```python
from build123d import *

# Parameters (mm, degrees)
SKETCH1_W           = 282.575
SKETCH1_H           = 384.175
SKETCH1_R           = 6.35
SKETCH1_R_2         = 1.5875
SKETCH1_W_2         = 127
SKETCH1_H_2         = 127
BOSS_EXTRUDE1_DEPTH = 2.54


with BuildPart() as part:
    # Sketch1 → Boss-Extrude1 (new body)
    with BuildSketch(Plane.XY):
        Rectangle(SKETCH1_W, SKETCH1_H)
        with Locations((-128.5875, 166.6875)):
            Circle(SKETCH1_R, mode=Mode.SUBTRACT)
        with Locations((-128.5875, -1.5875)):
            Circle(SKETCH1_R, mode=Mode.SUBTRACT)
        with Locations((-128.5875, -169.8625)):
            Circle(SKETCH1_R, mode=Mode.SUBTRACT)
        with Locations((128.5875, -1.5875)):
            Circle(SKETCH1_R, mode=Mode.SUBTRACT)
        with Locations((128.5875, 166.6875)):
            Circle(SKETCH1_R, mode=Mode.SUBTRACT)
        with Locations((128.5875, -169.8625)):
            Circle(SKETCH1_R, mode=Mode.SUBTRACT)
        with Locations((-80.175152311, 147.376386757)):
            Circle(SKETCH1_R_2, mode=Mode.SUBTRACT)
        with Locations((-80.175152311, 71.176386757)):
            Circle(SKETCH1_R_2, mode=Mode.SUBTRACT)
        with Locations((-80.175152311, -5.023613243)):
            Circle(SKETCH1_R_2, mode=Mode.SUBTRACT)
        with Locations((79.970650499, -5.395164494)):
            Circle(SKETCH1_R_2, mode=Mode.SUBTRACT)
        with Locations((79.970650499, 70.804835506)):
            Circle(SKETCH1_R_2, mode=Mode.SUBTRACT)
        with Locations((79.970650499, 147.004835506)):
            Circle(SKETCH1_R_2, mode=Mode.SUBTRACT)
        with Locations((-0.006402311, 49.2125)):
            Rectangle(SKETCH1_W_2, SKETCH1_H_2, mode=Mode.SUBTRACT)
    extrude(amount=BOSS_EXTRUDE1_DEPTH)


solid = part.part
```
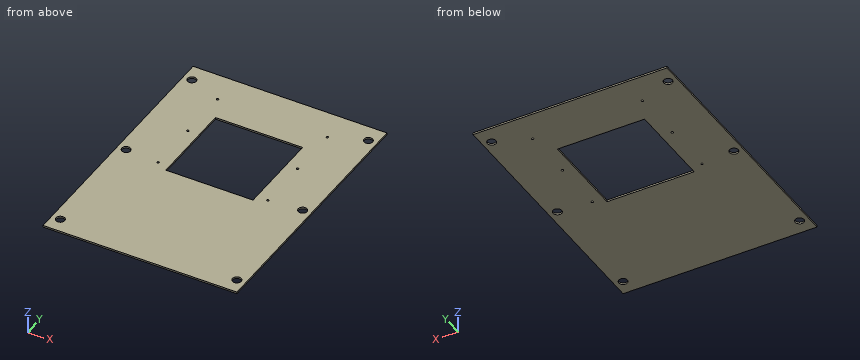
Design review of the part built by this model. Coordinates are the model's own, in mm. Coordinates: 2 decimals unless noted, no trailing zeros. Order: outer loops, then holes, each group sorted by start corner. A loop starts at its lowest first (then second) coordinate and runs counter-clockwise, first axis right, second up. Notation, with made-up numbers: (-2.5, 57.25) -> (24.5, 57.25) arc R17 ccw to (24.5, 87.25) -> close; hole circle Ø7 at (7.25, -13). An arc over 180 degrees is marked (long way). One line per item, written item: value. Start each with the question number.
Q1. Take a section at A-A, the plane x = 23.5. State the section outline as (y, z) points, then the cut area to 3 significant figures.
Q2. Take a section at B-B, the plane y = 91.5. State the section outline as (x, z) points, then the cut area to 3 significant figures.
Q3. For probe 1 along Y at (x, z) = (129, 1.5); probe 2 along X at (y, z) = (13, 1.85); probe 3 along Y at (x, z) = (-57, 2), list the stretches that pass through material, from the lowest coordinate up.
Q4. Take a section at C-C, the plane z = 1.4. Give the number of separate pieces and of enclosed holes in the cut face, then the cut area to 3 significant figures.
Q5. Insertion check: pin 1 Ø3 at (x, y) = (79.97, 70.8) entering from +Z. The pin has a flat end and moves straight along its axis. Give the tip position at first contact, or say it passes through.
Values follow:
1. outline: (-192.09, 0) -> (-14.29, 0) -> (-14.29, 2.54) -> (-192.09, 2.54) -> close; (112.71, 0) -> (192.09, 0) -> (192.09, 2.54) -> (112.71, 2.54) -> close
1. area: 653 mm2
2. outline: (-141.29, 0) -> (-63.51, 0) -> (-63.51, 2.54) -> (-141.29, 2.54) -> close; (63.49, 0) -> (141.29, 0) -> (141.29, 2.54) -> (63.49, 2.54) -> close
2. area: 395 mm2
3. probe 1: y = -192.09 to -176.2, -163.53 to -7.92, 4.75 to 160.35, 173.02 to 192.09
3. probe 2: x = -141.29 to -63.51, 63.49 to 141.29
3. probe 3: y = -192.09 to -14.29, 112.71 to 192.09
4. separate pieces: 1
4. enclosed holes: 13
4. area: 91,600 mm2
5. pin 1: passes through
